```python
from build123d import *

# Parameters (mm, degrees)
F0_R     = 12.5
F1_DEPTH = 50
F2_DEPTH = 25
F0_R_2   = 7.5
F3_DEPTH = 20


with BuildPart() as f1:
    # F0 (on Front) → F1 (new body)
    with BuildSketch(Plane.XZ):
        with BuildLine():
            Line((175.374043, 25), (50, 25))
            ThreePointArc((50, 25), (25, 0), (50, -25))
            Line((50, -25), (175.374043, -25))
            ThreePointArc((175.374043, -25), (200.374043, 0), (175.374043, 25))
        make_face()
        with Locations((50, 0)):
            Circle(F0_R, mode=Mode.SUBTRACT)
        with Locations((175.374043, 0)):
            Circle(F0_R, mode=Mode.SUBTRACT)
    extrude(amount=F1_DEPTH)

    # F0 (on Front) → F2 (join)
    with BuildSketch(Plane.XZ):
        with BuildLine():
            Line((225.374043, 50), (0, 50))
            ThreePointArc((0, 50), (-50, 0), (0, -50))
            Line((0, -50), (225.374043, -50))
            ThreePointArc((225.374043, -50), (275.374043, 0), (225.374043, 50))
        make_face()
        Circle(F0_R, mode=Mode.SUBTRACT)
        with BuildLine():
            ThreePointArc((50, -25), (25, 0), (50, 25))
            Line((50, 25), (175.374043, 25))
            ThreePointArc((175.374043, 25), (200.374043, 0), (175.374043, -25))
            Line((175.374043, -25), (50, -25))
        make_face(mode=Mode.SUBTRACT)
        with Locations((225.374043, 0)):
            Circle(F0_R, mode=Mode.SUBTRACT)
    extrude(amount=F2_DEPTH)

    # F0 (on Front) → F3 (join)
    with BuildSketch(Plane.XZ):
        Circle(F0_R)
        Circle(F0_R_2, mode=Mode.SUBTRACT)
        with Locations((225.374043, 0)):
            Circle(F0_R)
        with Locations((225.374043, 0)):
            Circle(F0_R_2, mode=Mode.SUBTRACT)
    extrude(amount=F3_DEPTH)


solid = f1.part
```
For this review, take the finished solid that the model builds, in its own axes (mm). A direction names the side the tool comes from. Round coordinates to 2 decimals unless told otherwise and drop trailing zeros. Write each loop counter-clockwise with the first axis right and the second up, starting at its lowest first coordinate (ties: lowest second). Pieces come first, ordered by that corner, then holes. Notation, with made-up numbers: (80, -38) - (103, -38) arc R31 cw to (103, -3) - close; hole circle Ø5 at (35.25, 2.25). An arc over 180 degrees is marked (long way). Write each question's results on one line, items separated by ' | '.
Item 1: Draft analysis for pull direction Z (two halves, no side actions). For faces 6 (the face through (114, -12, 50)), 7 (the face through (110, -25, 34)), 8 (the face through (217.88, -9.86, 0.33)), state which applies: pulls with the +Z half, pulls with the -Z half, needs draft (parallel to the pull), parting line crosses it, or undercut.
Calculated:
face 6: pulls with the +Z half | face 7: needs draft | face 8: undercut
Item 2: For faces 1 (the face through (112, -37, -25)), 2 (the face through (200.368, -37.325, -0.55)), 3 (the face through (25.006, -37.325, 0.55)), 4 (the face through (114, -37, 25)), 5 (the face through (0, -20, -8)), list the 3-axis set-ups (+Z, -Z, +X, -X, +Y, -Y) from which the entire face can be reached by the end or side of a thin tool; tool diameter is ignored.
Calculated:
face 1: -Z, +X, -X, -Y | face 2: +X, -Y | face 3: -X, -Y | face 4: +Z, +X, -X, -Y | face 5: -Y
Item 3: Take a section at D-D on y = -9.5. State the section outline as (x, z) points, then the cut area to 3 significant figures.
Calculated:
outline: (0, -50) - (225.37, -50) arc R50 ccw to (225.37, 50) - (0, 50) arc R50 ccw to start; hole circle Ø15 at (0, 0); hole circle Ø25 at (50, 0); hole circle Ø25 at (175.37, 0); hole circle Ø15 at (225.37, 0) | area: 29,100 mm^2
Item 4: Take a section at B-B on y = -28. State the section outline as (x, z) points.
Calculated:
outline: (50, -25) - (175.37, -25) arc R25 ccw to (175.37, 25) - (50, 25) arc R25 ccw to start; hole circle Ø25 at (50, 0); hole circle Ø25 at (175.37, 0)
Item 5: To check wall thickness, follow line 1 along Z through (x, y) = (0, -21.15); line 2 along X through (y, z) = (-3.5, -2); line 3 along X through (y, z) = (-17.5, 8). State the ranges of each line that lie inside material, in increasing order. Write a range as from..to.
Calculated:
line 1: z = -50..-12.5, 12.5..50 | line 2: x = -49.96..-7.23, 7.23..37.66, 62.34..163.04, 187.71..218.15, 232.6..275.33 | line 3: x = -49.36..40.4, 59.6..165.77, 184.98..274.73
Item 6: For pin 1 (22.5 mm diameter, centred on x = 225.37, z = 0, fed in from +Y); pin 2 (10 mm diameter, centred on y = -17.5, z = 39.5, fed in from +X); pin 3 (7.5 mm diameter, centred on x = 136, y = -43.5, fed in from +Z); pin 4 (20 mm diameter, centred on x = 5, z = -3.5, fed in from -Y), all flat-tipped, find the tip position at first contact; note any pin that passes through.
Calculated:
pin 1: stops at y = 0 | pin 2: stops at x = 261.56 | pin 3: stops at z = 25 | pin 4: stops at y = -25
Item 7: Take a section at A-A on z = 0. Count the separate pieces of the cut face and the enclosed holes in it, then the cut area to 3 significant figures.
Calculated:
separate pieces: 5 | enclosed holes: 0 | area: 9,170 mm^2
Item 8: Take a section at C-C on x = 45. State the section outline as (y, z) points.
Calculated:
outline: (-50, -24.49) - (-25, -24.49) - (-25, -50) - (0, -50) - (0, -11.46) - (-50, -11.46) - close; (-50, 11.46) - (0, 11.46) - (0, 50) - (-25, 50) - (-25, 24.49) - (-50, 24.49) - close
